from build123d import *

# Parameters (mm, degrees)
BOSS_EXTRU_1_DEPTH      = 3
ESQUISSE2_R             = 2
ENL_V_MAT_EXTRU_1_DEPTH = 3


with BuildPart() as part:
    # Esquisse1 → Boss.-Extru.1 (new body)
    with BuildSketch(Plane.XY):
        with BuildLine():
            Line((0, 5), (30, 5))
            ThreePointArc((30, 5), (35, 0), (30, -5))
            Line((30, -5), (0, -5))
            ThreePointArc((0, -5), (-5, 0), (0, 5))
        make_face()
    extrude(amount=BOSS_EXTRU_1_DEPTH)

    # Esquisse2 → Enlèv. mat.-Extru.1 (cut)
    with BuildSketch(Plane.XY.offset(3)):
        with Locations((32.217323413, 0)):
            Circle(ESQUISSE2_R)
    extrude(amount=-ENL_V_MAT_EXTRU_1_DEPTH, mode=Mode.SUBTRACT)


solid = part.part
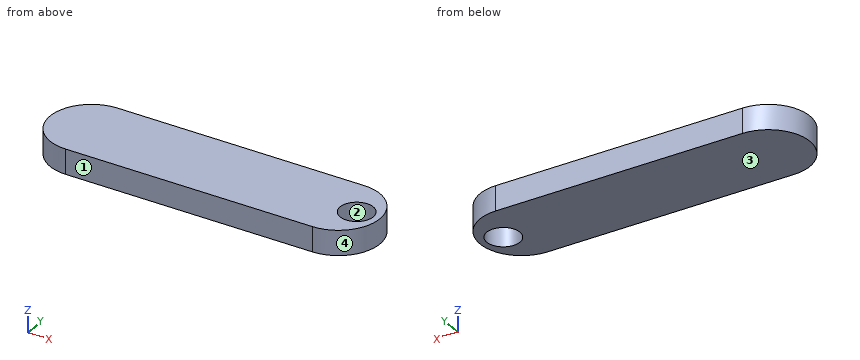
Can you work these out from the model? Positions are in its coordinate system, mm. Face numbers are marked on the shaded views. Coordinates: 2 decimals unless noted, no trailing zeros. Loops run counter-clockwise (first coordinate to the right, second up) from the corner with the lowest first, then second, coordinate; pieces in that order, holes last. Notation, with made-up numbers: M 83.5,-26.5 L 118.5,-26.5 A13 ccw 118.5,-20.5 Z; hole C -10,7.5 d11. An arc over 180 degrees is marked long. Return JSON: item names as keys, results as strings. Group by question number.
Item 1: If I drill on L1, parallel to Y at x = 32.5, z = 2.8; L2, parallel to X at y = -0.5, z = 2.45; L3, parallel to Y at x = 32, z = 0.8, over which ranges is the centre line in solid material (lowest first)? Write a range as from..to.
Item 2: Imagine slicing it at D-D (x = -1). Please give me the cut outline in (y, z).
Item 3: Thinking about a two-plate mould opening in Y: for the marked faces 1, 2, 3 and 4, which applies, released by +Y, released by -Y, zero draft, split by the parting line, or undercut?
Item 4: Imagine slicing it at B-B (x = 32.5). Please give me the cut outline in (y, z).
Item 5: I'm going to push a flat-ended pin straight in: pin 1 Ø4.5 at (x, y) = (32.22, 0) entering from -Z. Where does the tip first touch, or does it pass through?
Item 6: Imagine slicing it at A-A (z = 1.3). Please give me the cut outline in (x, y), and give its area (3 significant figures).
Item 7: Imagine slicing it at C-C (y = 1). Please give me the cut outline in (x, z).
Verdict:
{
 "1": {"L1": "y = -4.33..-1.98, 1.98..4.33", "L2": "x = -4.97..30.28, 34.15..34.97", "L3": "y = -4.58..-1.99, 1.99..4.58"},
 "2": {"outline": "M -4.9,0 L 4.9,0 L 4.9,3 L -4.9,3 Z"},
 "3": {"face 1": "released by -Y", "face 2": "undercut", "face 3": "zero draft", "face 4": "split by the parting line"},
 "4": {"outline": "M -4.33,0 L -1.98,0 L -1.98,3 L -4.33,3 Z; M 1.98,0 L 4.33,0 L 4.33,3 L 1.98,3 Z"},
 "5": {"pin 1": "stops at z = 0"},
 "6": {"outline": "M 0,-5 L 30,-5 A5 ccw 30,5 L 0,5 A5 ccw Z; hole C 32.22,0 d4", "area": "366 mm^2"},
 "7": {"outline": "M -4.9,0 L 30.49,0 L 30.49,3 L -4.9,3 Z; M 33.95,0 L 34.9,0 L 34.9,3 L 33.95,3 Z"}
}
